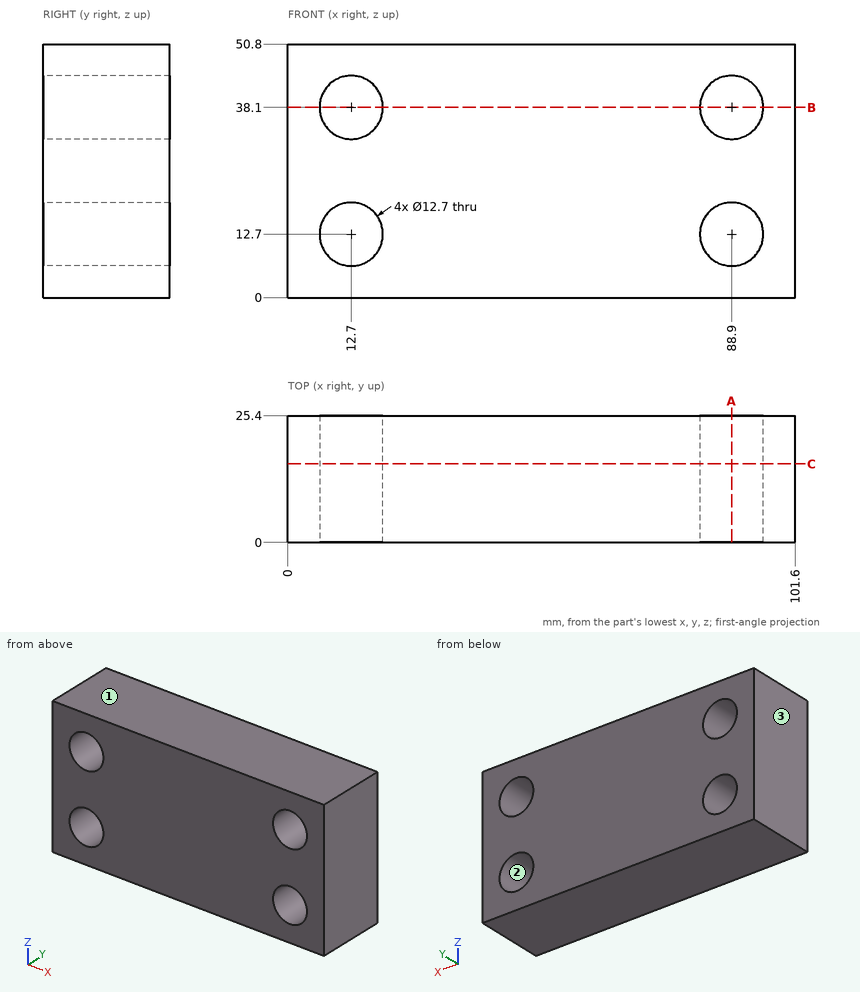
Could you check a few things on this drawing? It's one solid part, dimensions in mm from its lowest x, y, z. Coordinates: 2 decimals unless noted, no trailing zeros. Order: outer loops, then holes, each group sorted by start corner. A loop starts at its lowest first (then second) coordinate and runs counter-clockwise, first axis right, second up.
1) Imagine slicing it at A-A on x = 88.9. List the corners of the cut face in (y, z) for me.
2) We'd pull the mould along Z, two halves only. Please class the marked faces 1, 2 and 3: +Z half, -Z half, draft (parallel to the pull), parting line (faces both ways), or undercut.
3) I need wall thicknesses on line 1 (Z direction, x = 12.7, y = 17.5); line 2 (X direction, y = 20.25, z = 12.5); line 3 (X direction, y = 13.5, z = 16). Which ranges of each line are inside material? Lowest first, please.
4) Imagine slicing it at C-C on y = 15.75. List the corners of the cut face in (x, z) for me.
5) Imagine slicing it at B-B on z = 38.1. List the corners of the cut face in (x, y) for me.
Response values:
1. outline: (0, 0) - (25.4, 0) - (25.4, 6.35) - (0, 6.35) - close; (0, 19.05) - (25.4, 19.05) - (25.4, 31.75) - (0, 31.75) - close; (0, 44.45) - (25.4, 44.45) - (25.4, 50.8) - (0, 50.8) - close
2. face 1: +Z half
2. face 2: undercut
2. face 3: draft
3. line 1: z = 0 to 6.35, 19.05 to 31.75, 44.45 to 50.8
3. line 2: x = 0 to 6.35, 19.05 to 82.55, 95.25 to 101.6
3. line 3: x = 0 to 7.27, 18.13 to 83.47, 94.33 to 101.6
4. outline: (0, 0) - (101.6, 0) - (101.6, 50.8) - (0, 50.8) - close; hole circle Ø12.7 at (12.7, 12.7); hole circle Ø12.7 at (12.7, 38.1); hole circle Ø12.7 at (88.9, 12.7); hole circle Ø12.7 at (88.9, 38.1)
5. outline: (0, 0) - (6.35, 0) - (6.35, 25.4) - (0, 25.4) - close; (19.05, 0) - (82.55, 0) - (82.55, 25.4) - (19.05, 25.4) - close; (95.25, 0) - (101.6, 0) - (101.6, 25.4) - (95.25, 25.4) - close
